from build123d import *

# Parameters (mm, degrees)
SKETCH4_R          = 1.6
CUT_EXTRUDE1_DEPTH = 2
CUT_EXTRUDE2_REACH = 15.49
CIRPATTERN1_COUNT  = 3
FILLET1_R          = 0.1


with BuildPart() as part:
    # Sketch2 → Revolve1 (revolve)
    with BuildSketch(Plane(origin=(0, 0, 0), x_dir=(0, 0, -1), z_dir=(1, 0, 0))):
        with BuildLine():
            Line((2.45, 0), (3.25, 0))
            Line((3.25, 0), (3.25, 1.1))
            Line((3.25, 1.1), (3.35, 1.1))
            ThreePointArc((3.35, 1.1), (4.587436867, 1.612563133), (5.1, 2.85))
            Line((5.1, 2.85), (5.1, 7.85))
            ThreePointArc((5.1, 7.85), (4.587436867, 9.087436867), (3.35, 9.6))
            Line((3.35, 9.6), (2.45, 9.6))
            Line((2.45, 9.6), (2.45, 11.4))
            Line((2.45, 11.4), (0, 11.4))
            Line((0, 11.4), (0, 8.5))
            Line((0, 8.5), (2.45, 8.5))
            Line((2.45, 8.5), (2.45, 0))
        make_face()
    revolve(axis=Axis((0, 0, 0), (0, 1, 0)))

    # Sketch4 → Cut-Extrude1 (cut)
    with BuildSketch(Plane(origin=(0, 11.4, 0), x_dir=(1, 0, 0), z_dir=(0, 1, 0))):
        with Locations(Location((0, 0, 0), (0, 0, 270))):
            Circle(SKETCH4_R)
    extrude(amount=-CUT_EXTRUDE1_DEPTH, mode=Mode.SUBTRACT)

    # Sketch5 → Cut-Extrude2 (cut, up to next)
    with BuildSketch(Plane(origin=(0, 11.4, 0), x_dir=(1, 0, 0), z_dir=(0, 1, 0)), mode=Mode.PRIVATE) as cut_extrude2_sk1:
        with BuildLine():
            Line((-1.547048989, -0.408214924), (-0.42, 0.242487113))
            Line((-0.42, 0.242487113), (-0.42, 1.543891188))
            ThreePointArc((-0.42, 1.543891188), (-1.385640646, 0.8), (-1.547048989, -0.408214924))
        make_face()
    cut_extrude2_tool1 = extrude(cut_extrude2_sk1.sketch, amount=-CUT_EXTRUDE2_REACH, mode=Mode.PRIVATE) & part.part
    cut_extrude2 = cut_extrude2_tool1.solids().sort_by_distance((-0.969614, 11.4, -0.559807))[0]
    add(cut_extrude2, mode=Mode.SUBTRACT)

    # CirPattern1: Cut-Extrude2 ×3 about axis
    cirpattern1_axis = Axis((0, 0, 0), (0, 1, 0))
    for i in range(1, CIRPATTERN1_COUNT):
        add(cut_extrude2.rotate(cirpattern1_axis, i * 360 / CIRPATTERN1_COUNT), mode=Mode.SUBTRACT)

    # Fillet1
    fillet1_edges = [part.edges().sort_by_distance(p)[0] for p in [
        (0, 11.4, 2.45),
    ]]
    fillet(fillet1_edges, radius=FILLET1_R)


solid = part.part
Can you work these out from the model? Positions are in its coordinate system, mm. A direction names the side the tool comes from. Round coordinates to 2 decimals unless told otherwise and drop trailing zeros. Write each loop counter-clockwise with the first axis right and the second up, starting at its lowest first coordinate (ties: lowest second). Pieces come first, ordered by that corner, then holes. Notation, with made-up numbers: M 69,47.5 L 84,47.5 A17 cw 84,56.5 Z; hole C -33.5,59 d11. An arc over 180 degrees is marked long. Use CSV: the item, a comma, the result in double quotes.
(1) Imagine slicing it at A-A (z = 0). Count the separate pieces of the cut face and the enclosed holes in it, plus the area to 3 significant figures.
Check values:
separate pieces,"3"
enclosed holes,"0"
area,"50.6 mm^2"
(2) I'm going to push flat-ended pins straight in: pin 1 (1.5 mm diameter, centred on x = 2, y = 6.5, fed in from +Z); pin 2 (1 mm diameter, centred on y = 9, z = -1, fed in from -X); pin 3 (4 mm diameter, centred on x = 0, z = 0, fed in from -Y). Where does each tip first touch, or does it pass through?
Check values:
pin 1,"z = 4.94"
pin 2,"x = -4.89"
pin 3,"y = 8.5"
(3) Imagine slicing it at C-C (y = 10.75). Write out the boundary of the cut face in (x, z).
Check values:
outline,"C 0,0 d4.9; hole C 0,0 d3.2"
(4) Imagine slicing it at B-B (y = 4.75). Write out the boundary of the cut face in (x, z).
Check values:
outline,"C 0,0 d10.2; hole C 0,0 d4.9"
(5) On a 3-axis mill with a long thin cutter (end or side, diameter ignored), from which of +Z, -Z, +X, -X, +Y, -Y can I reach the whole of each face in a straight line? I mean faces 1 (the flat face through (0, 9.4, 0)), 2 (the flat face through (0.98, 8.96, 0.08)), 3 (the flat face through (0, 8.5, 0)). Say none if no direction works.
Check values:
face 1,"+Y"
face 2,"+Y, -Y"
face 3,"-Y"
(6) I need wall thicknesses on line 1 along X through (y, z) = (3.25, 0); line 2 along X through (y, z) = (9.9, 0); line 3 along X through (y, z) = (8.75, -1). Which ranges of each line are inside material? Lowest first, please.
Check values:
line 1,"-5.1 to -2.45, 2.45 to 5.1"
line 2,"-2.45 to -1.6, 1.6 to 2.45"
line 3,"-4.75 to -1.25, -0.42 to 0.42, 1.25 to 4.75"
(7) We'd pull the mould along X, two halves only. Please class faces 4 (the cylindrical face through (2.4, 10.5, 0.5)), 5 (the flat face through (0, 11.4, -2)), 6 (the flat face through (0.42, 9, -1)), 7 (the flat face through (0.571, 8.956, 0.815)): +X half, -X half, draft (parallel to the pull), parting line (faces both ways), or undercut.
Check values:
face 4,"parting line"
face 5,"draft"
face 6,"undercut"
face 7,"undercut"
